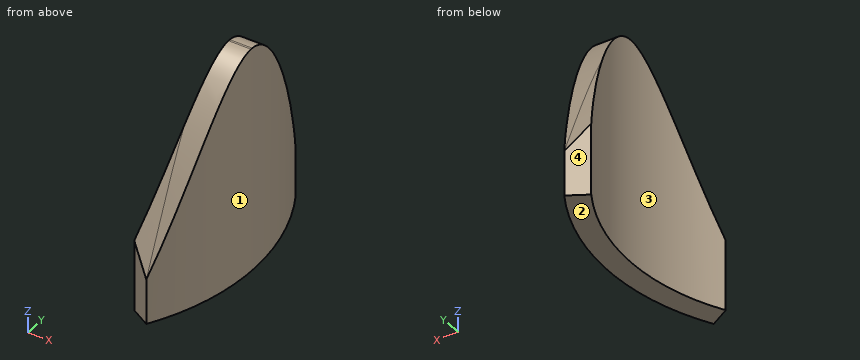
from build123d import *

# Parameters (mm, degrees)
F1_DEPTH = 12.7
F3_DEPTH = 6.35


# Not quite as in the source:
# - a feature names something its author has since deleted; it is built from what else it names


with BuildPart() as f1:
    # F0 (on Top) → F1 (new body)
    with BuildSketch(Plane.XY):
        with BuildLine():
            Line((-1.099852253, -12.0650000057), (0, -12.7))
            ThreePointArc((0, -12.7), (1.7014773719, -6.35), (0, 0))
            Line((0, 0), (-1.099852253, -0.6349999943))
            ThreePointArc((-1.099852253, -0.6349999943), (0.4314773832, -6.35), (-1.099852253, -12.0650000057))
        make_face()
    extrude(amount=F1_DEPTH)

    # F2 (on Right) → F3 (cut, symmetric)
    with BuildSketch(Plane.YZ):
        with BuildLine():
            Line((0, 12.7), (-6.259501017, 12.7))
            add(Edge.make_bspline(
                [(0, 2.54), (-2.0835692993, 7.5354677351), (-4.1744975267, 12.6135905998), (-6.259501017, 12.7)],
                knots=[0, 0, 0, 0, 0.4917268941, 0.4917268941, 0.4917268941, 0.4917268941], degree=3))
            Line((0, 2.54), (0, 12.7))
        make_face()
        with BuildLine():
            add(Edge.make_bspline(
                [(-6.259501017, 12.7), (-6.2953843519, 12.7014871234), (-6.331265932, 12.7014957456), (-6.3671456895, 12.7)],
                knots=[0.4917268941, 0.4917268941, 0.4917268941, 0.4917268941, 0.5001896141, 0.5001896141, 0.5001896141, 0.5001896141], degree=3))
            Line((-6.3671456895, 12.7), (-6.259501017, 12.7))
        make_face()
        with BuildLine():
            add(Edge.make_bspline(
                [(-6.3671456895, 12.7), (-8.4862132407, 12.6116608867), (-10.5989234677, 7.2759161441), (-12.7, 2.54)],
                knots=[0.5001896141, 0.5001896141, 0.5001896141, 0.5001896141, 1, 1, 1, 1], degree=3))
            Line((-6.3671456895, 12.7), (-12.7, 12.7))
            Line((-12.7, 12.7), (-12.7, 2.54))
        make_face()
    extrude(amount=F3_DEPTH, both=True, mode=Mode.SUBTRACT)


solid = f1.part
Verification items for the finished model (mm, model axes). Face numbers are marked on the shaded views. Coordinates: 2 decimals unless noted, no trailing zeros. Write each loop counter-clockwise with the first axis right and the second up, starting at its lowest first coordinate (ties: lowest second). Pieces come first, ordered by that corner, then holes. Notation, with made-up numbers: (3, -1.5) -> (36, -1.5) arc R6 ccw to (36, 2.5) -> close; hole circle Ø10 at (11.25, 37.25). An arc over 180 degrees is marked (long way). One line per item, written item: value. Start each with the question number.
Q1. Go/stop test with flat-tipped pins: P1, Ø3, axis at y = -9, z = 2, coming from the -X side; P2, Ø1, axis at x = 1, y = -9, coming from the +Z side; P3, Ø1, axis at x = 0, y = -8, coming from the +Z side. Record where each tip stops, or that it passes through.
Q2. Thickness scan on L1, parallel to Y at x = -0.5, z = 2.5; L2, parallel to Z at x = 0.85, y = -5.25; L3, parallel to Z at x = 0, y = -0.75. Record the ranges inside material, lowest first. Write a range as from..to.
Q3. Mould release check, pull along Y, two halves, no side actions. Record for the marked faces 1, 2, 3 and 4: pulls with the +Y half, pulls with the -Y half, needs draft (parallel to the pull), parting line crosses it, or undercut.
Q4. Cross-section at A-A on z = 2. Enter the section's corners in (x, y) (3 decimals).
Checked values:
1. P1: stops at x = -0.35
1. P2: stops at z = 11.06
1. P3: stops at z = 12.05
2. L1: y = -12.41..-10.87, -1.83..-0.29
2. L2: z = 0..12.29
2. L3: z = 0..4.33
3. face 1: parting line crosses it
3. face 2: needs draft
3. face 3: undercut
3. face 4: pulls with the +Y half
4. outline: (-1.1, -12.065) -> (0, -12.7) arc R12.7 ccw to (0, 0) -> (-1.1, -0.635) arc R11.43 cw to start
